from build123d import *


with BuildPart() as part:
    # Sketch1 → Revolve-Thin1 (revolve)
    with BuildSketch(Plane.XY):
        Polygon((-177.698412698, 15), (-152.698412698, 15), (-62.698412698, 15), (-62.698412698, 20), (-29.728412698, 20), (-29.728412698, 15), (-9.728412698, 15), (-9.728412698, 20), (23.241587302, 20), (23.241587302, 15), (43.241587302, 15), (43.241587302, 20), (76.211587302, 20), (76.211587302, 15), (192.237786857, 15), (497.301587302, 15), (522.301587302, 15), (522.301587302, 5), (497.301587302, 5), (192.237786857, 5), (66.211587302, 5), (66.211587302, 10), (53.241587302, 10), (53.241587302, 5), (13.241587302, 5), (13.241587302, 10), (0.271587302, 10), (0.271587302, 5), (-39.728412698, 5), (-39.728412698, 10), (-52.698412698, 10), (-52.698412698, 5), (-152.698412698, 5), (-177.698412698, 5), align=None)
    revolve(axis=Axis((-114.603174603, 0, 0), (1, 0, 0)))


solid = part.part
CAD build for the part. Positions are in the model's coordinates, mm. A direction names the side the tool comes from. Give positions to 0.01 mm unless a question says otherwise; leave off trailing zeros. Write each loop counter-clockwise with the first axis right and the second up, starting at its lowest first coordinate (ties: lowest second). Pieces come first, ordered by that corner, then holes. Notation, with made-up numbers: (-21.5, 2.25) - (11.5, 2.25) arc R21 ccw to (11.5, 8.25) - close; hole circle Ø1 at (-32.75, -0.5). An arc over 180 degrees is marked (long way). Answer as CSV lines item,"result".
Q1. Drill centre lines: line 1 (X direction, y = 17.5, z = 8); line 2 (X direction, y = 8, z = 3.5); line 3 (Z direction, x = 7, y = 0). Where is each one in solid material? Low to high. Write a range as from..to.
Result set:
line 1,"-62.7..-29.73, -9.73..23.24, 43.24..76.21"
line 2,"-177.7..-52.7, -39.73..0.27, 13.24..53.24, 66.21..522.3"
line 3,"-20..-10, 10..20"
Q2. 3-axis set-ups, long thin cutter, end or side, ignore diameter. For faces 1 (the face through (-121.003, -14.985, 0.66)), 2 (the face through (59.64, -2.17, -9.76)), 3 (the face through (76.212, 3, 15)), 4 (the face through (-177.698, 4, 4)), 5 (the face through (6.987, -4.336, -19.524)): which of +Z, -Z, +X, -X, +Y, -Y reach the whole face in a straight line?
Result set:
face 1,"-X"
face 2,"none"
face 3,"+X"
face 4,"+Z, -Z, -X, +Y, -Y"
face 5,"+X, -X"
Q3. Pull direction X, two halves, no side cores. Call faces 6 (the face through (522.302, -4, 4)), 7 (the face through (-62.698, -3, 15)), 8 (the face through (-39.728, -2, 5)): released by +X, released by -X, zero draft, split by the parting line, or undercut.
Result set:
face 6,"released by +X"
face 7,"released by -X"
face 8,"undercut"
Q4. Flat gauge pins, fed straight in: pin 1 Ø23 at (y, z) = (0, 0) entering from -X; pin 2 Ø3 at (y, z) = (-16, 13) entering from -X; pin 3 Ø10 at (x, z) = (44.5, 12.5) entering from +Y; pin 4 Ø12 at (x, z) = (-88.5, 12.5) entering from +Y. Where does each tip first touch, or does it go through?
Result set:
pin 1,"x = -177.7"
pin 2,"x = -62.7"
pin 3,"y = 18.54"
pin 4,"y = 13.52"
Q5. Band-saw the part on A-A (x = 321). Give the cut face in (y, z).
Result set:
outline,"circle Ø30 at (0, 0); hole circle Ø10 at (0, 0)"
